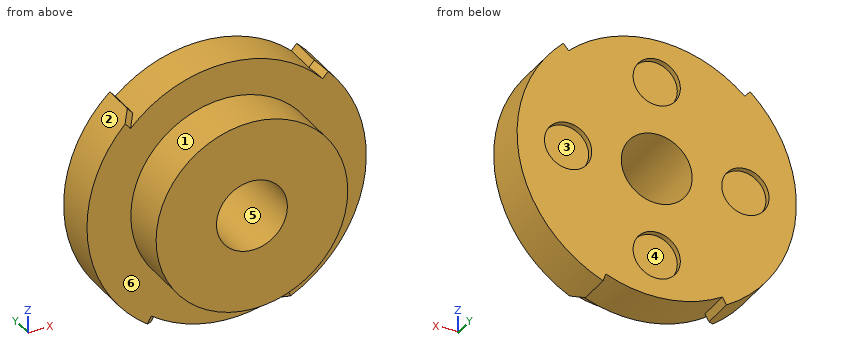
```python
from build123d import *

# Parameters (mm, degrees)
F0_R      = 236.347
F1_DEPTH  = 76.2
F2_R      = 162.179
F3_DEPTH  = 82.55
F5_DEPTH  = 139.7
F6_SIZE   = 19.05
F7_SIZE   = 19.05
F8_SIZE   = 19.05
F9_SIZE   = 19.05
F10_R     = 40
F11_DEPTH = 10
F12_R     = 60
F13_DEPTH = 550


with BuildPart() as f1:
    # F0 (on Front) → F1 (new body)
    with BuildSketch(Plane.XZ):
        Circle(F0_R)
    extrude(amount=F1_DEPTH)

    # F2 (on face) → F3 (join)
    with BuildSketch(Plane.XZ.offset(76.2)):
        Circle(F2_R)
    extrude(amount=F3_DEPTH)

    # F4 (on face) → F5 (cut)
    with BuildSketch(Plane(origin=(0, 0, 0), x_dir=(-1, 0, 0), z_dir=(0, 1, 0))):
        with BuildLine():
            Line((-184.812798, 205.255406), (-148.926726, 165.399886))
            ThreePointArc((-148.926726, 165.399886), (0, 222.5675), (148.926726, 165.399886))
            Line((148.926726, 165.399886), (183.385925, 203.670703))
            Line((183.385925, 203.670703), (0, 288.642466))
            Line((0, 288.642466), (-184.812798, 205.255406))
        make_face()
        with BuildLine():
            Line((138.952692, -240.673122), (111.28375, -192.749109))
            ThreePointArc((111.28375, -192.749109), (14.086917, -222.121253), (-86.041814, -205.263485))
            Line((-86.041814, -205.263485), (-123.598595, -308.449893))
            Line((-123.598595, -308.449893), (23.055677, -307.586295))
            Line((23.055677, -307.586295), (138.952692, -240.673122))
        make_face()
    extrude(amount=-F5_DEPTH, mode=Mode.SUBTRACT)

    # F6
    f6_edges = [f1.edges().sort_by_distance(p)[0] for p in [
        (88.400791, -76.2, -211.744722),
    ]]
    chamfer(f6_edges, length=F6_SIZE)

    # F7
    f7_edges = [f1.edges().sort_by_distance(p)[0] for p in [
        (-114.728625, -76.2, -198.715808),
    ]]
    chamfer(f7_edges, length=F7_SIZE)

    # F8
    f8_edges = [f1.edges().sort_by_distance(p)[0] for p in [
        (153.536869, -76.2, 170.519968),
    ]]
    chamfer(f8_edges, length=F8_SIZE)

    # F9
    f9_edges = [f1.edges().sort_by_distance(p)[0] for p in [
        (-153.536869, -76.2, 170.519968),
    ]]
    chamfer(f9_edges, length=F9_SIZE)

    # F10 (on face) → F11 (cut)
    with BuildSketch(Plane(origin=(0, 0, 0), x_dir=(-1, 0, 0), z_dir=(0, 1, 0))):
        with Locations((0, 150)):
            Circle(F10_R)
        with Locations((-150, 0)):
            Circle(F10_R)
        with Locations((0, -150)):
            Circle(F10_R)
        with Locations((150, 0)):
            Circle(F10_R)
    extrude(amount=-F11_DEPTH, mode=Mode.SUBTRACT)

    # F12 (on face) → F13 (cut)
    with BuildSketch(Plane.XZ.offset(158.75)):
        Circle(F12_R)
    extrude(amount=-F13_DEPTH, mode=Mode.SUBTRACT)


solid = f1.part
```
Could you check a few things on this model? Use its own coordinates, in mm. Face numbers are marked on the shaded views. A direction names the side the tool comes from. Coordinates: 2 decimals unless noted, no trailing zeros. Order: outer loops, then holes, each group sorted by start corner. A loop starts at its lowest first (then second) coordinate and runs counter-clockwise, first axis right, second up. Notation, with made-up numbers: M -30,-31.5 L -14,-31.5 A25 cw -14,-15.5 Z; hole C -9,3.25 d7. An arc over 180 degrees is marked long. Use one line per item in the form item = value. Start each with the question number.
1. Suppose I cut it at C-C on y = -17. Write out the boundary of the cut face in (x, z) (1 decimal), then the cut area to 3 significant figures.
2. Suppose I cut it at A-A on x = 0. Write out the boundary of the cut face in (y, z).
3. Please list where these lines run through material, in increasing order: line 1 (Z direction, x = 0, y = -4.5); line 2 (X direction, y = -113.5, z = -2); line 3 (Y direction, x = 65.5, z = -169.5).
4. Suppose I cut it at D-D on x = 70.5. Write out the boundary of the cut face in (y, z), then the cut area to 3 significant figures.
5. On a 3-axis mill with a long thin cutter (end or side, diameter ignored), from which of +Z, -Z, +X, -X, +Y, -Y can I reach the whole of each face in a straight line? I mean the marked faces 4, 5 and 6. Say none if no direction works.
6. Suppose I cut it at B-B on z = 0. Write out the boundary of the cut face in (x, y).
7. For pin 1 (24 mm diameter, centred on x = 1, z = -139.5, fed in from +Y); pin 2 (5 mm diameter, centred on y = -135.5, z = -24.5, fed in from -X); pin 3 (6 mm diameter, centred on x = -26.5, y = -128, fed in from -Z), each with a flat end and sliding along its axis, tell me the tip position at first contact or that it passes through.
8. We'd pull the mould along X, two halves only. Please class the marked faces 1, 2 and 3: +X half, -X half, draft (parallel to the pull), parting line (faces both ways), or undercut.
Geometry says:
q1.outline = M -158.1,175.6 A236.3 ccw -118.2,-204.7 L -111.3,-192.7 A222.6 ccw 86,-205.3 L 90.8,-218.2 A236.3 ccw 158.1,175.6 L 148.9,165.4 A222.6 ccw -148.9,165.4 Z; hole C 0,0 d120
q1.area = 157,000 mm^2
q2.outline = M -158.75,-162.18 L -76.2,-162.18 L -76.2,-222.57 L 0,-222.57 L 0,-190 L -10,-190 L -10,-110 L 0,-110 L 0,-60 L -158.75,-60 Z; M -158.75,60 L 0,60 L 0,110 L -10,110 L -10,190 L 0,190 L 0,222.57 L -76.2,222.57 L -76.2,162.18 L -158.75,162.18 Z
q3.line_1 = -222.57 to -190, -110 to -60, 60 to 110, 190 to 222.57
q3.line_2 = -162.17 to -59.97, 59.97 to 162.17
q3.line_3 = -76.2 to 0
q4.outline = M -158.75,-146.05 L -76.2,-146.05 L -76.2,-211.11 L 0,-211.11 L 0,211.11 L -76.2,211.11 L -76.2,146.05 L -158.75,146.05 Z
q4.area = 56,300 mm^2
q5.face_4 = +Y
q5.face_5 = +Y, -Y
q5.face_6 = -Y
q6.outline = M -236.35,-76.2 L -162.18,-76.2 L -162.18,-158.75 L -60,-158.75 L -60,0 L -110,0 L -110,-10 L -190,-10 L -190,0 L -236.35,0 Z; M 60,-158.75 L 162.18,-158.75 L 162.18,-76.2 L 236.35,-76.2 L 236.35,0 L 190,0 L 190,-10 L 110,-10 L 110,0 L 60,0 Z
q7.pin_1 = -10
q7.pin_2 = -160.68
q7.pin_3 = -160.47
q8.face_1 = parting line
q8.face_2 = -X half
q8.face_3 = undercut
